Check sheet for the modelled part. Datum: model origin and axes. Units: mm. A direction names the side the tool comes from. Coordinates: 2 decimals unless noted, no trailing zeros. Loops run counter-clockwise (first coordinate to the right, second up) from the corner with the lowest first, then second, coordinate; pieces in that order, holes last. Notation, with made-up numbers: (0, 11) - (58, 11) arc R31 ccw to (58, 38) - close; hole circle Ø5 at (87, -0.5). An arc over 180 degrees is marked (long way). Write each question's results on one line, items separated by ' | '. Start each with the question number.
1. Cross-section at A-A (y = 8.5). Record the cut outline in (x, z), and give its area (3 significant figures).
2. Tool access check on faces 4 (the face through (6, 13, 9)), 5 (the face through (-2.82, -5.02, 8.87)), 6 (the face through (-6, 17.7, 9)), 7 (the face through (-16.55, -5.52, 3.96)). Record the directions out of +Z, -Z, +X, -X, +Y, -Y that give a thin tool (end or side, any length) a straight path to the whole face; none if there is none.
3. Draft check along X on faces 1 (the face through (0, -4.796, 9)), 2 (the face through (-7.16, 9.726, 8.874)), 3 (the face through (-4.808, 0, 9)). Enter one of: released by +X, released by -X, zero draft, split by the parting line, or undercut.
4. Cross-section at B-B (x = 5). Record the cut outline in (y, z), and give its area (3 significant figures).
5. Gauge pin test, flat ends, axial feed: P1, Ø4, axis at y = -0.7, z = 5.25, coming from the +X side; P2, Ø1.5, axis at y = -5, z = 2.5, coming from the +X side; P3, Ø3, axis at y = -6.7, z = 5.25, coming from the -X side. Record the tip position at first contact, or that the pin passes through.
6. Thickness scan on line 1 (Y direction, x = -15.5, z = 5.25); line 2 (X direction, y = -5.5, z = 2); line 3 (Y direction, x = -5.25, z = 2.75). Record the ranges inside material, lowest first. Write a range as [from, to].
```python
from build123d import *

# Parameters (mm, degrees)
BOSS_EXTRUDE1_DEPTH = 18
SKETCH2_R           = 1.75
CUT_EXTRUDE1_DEPTH  = 7


with BuildPart() as part:
    # Sketch1 → Boss-Extrude1 (new body)
    with BuildSketch(Plane.XY):
        with BuildLine():
            Line((7.941784918, -13), (7.941784918, -17.7))
            Line((7.941784918, -17.7), (-20, -17.7))
            Line((-20, -17.7), (-20, 17.699847501))
            Line((-20, 17.699847501), (7.941784918, 17.699847501))
            Line((7.941784918, 17.699847501), (7.941784918, 13))
            Line((7.941784918, 13), (6.333126718, 13))
            Line((6.333126718, 13), (5.317126718, 13))
            Line((5.317126718, 13), (4.287512407, 13))
            ThreePointArc((4.287512407, 13), (3.333616586, 12.604883414), (2.9385, 11.650987593))
            Line((2.9385, 11.650987593), (2.9385, 11.539212407))
            ThreePointArc((2.9385, 11.539212407), (3.333616586, 10.585316586), (4.287512407, 10.1902))
            Line((4.287512407, 10.1902), (6.476788598, 10.1902))
            ThreePointArc((6.476788598, 10.1902), (7.154992901, 9.736757749), (6.995146796, 8.93674514))
            Line((6.995146796, 8.93674514), (3.686383353, 5.635543623))
            ThreePointArc((3.686383353, 5.635543623), (2.754473742, 5.014017446), (1.655778399, 4.7958))
            Line((1.655778399, 4.7958), (-1.655778399, 4.7958))
            ThreePointArc((-1.655778399, 4.7958), (-2.754473742, 5.014017446), (-3.686383353, 5.635543623))
            Line((-3.686383353, 5.635543623), (-6.995146796, 8.93674514))
            ThreePointArc((-6.995146796, 8.93674514), (-7.154992901, 9.736757749), (-6.476788598, 10.1902))
            Line((-6.476788598, 10.1902), (-4.287512407, 10.1902))
            ThreePointArc((-4.287512407, 10.1902), (-3.333616586, 10.585316586), (-2.9385, 11.539212407))
            Line((-2.9385, 11.539212407), (-2.9385, 11.650987593))
            ThreePointArc((-2.9385, 11.650987593), (-3.333616586, 12.604883414), (-4.287512407, 13))
            Line((-4.287512407, 13), (-5.317126718, 13))
            Line((-5.317126718, 13), (-6.333126718, 13))
            Line((-6.333126718, 13), (-9.550465633, 13))
            Line((-9.550465633, 13), (-10.564722121, 12.999847763))
            ThreePointArc((-10.564722121, 12.999847763), (-12.294654751, 12.29465435), (-12.999847757, 10.564721553))
            Line((-12.999847757, 10.564721553), (-13, 9.550422515))
            Line((-13, 9.550422515), (-13, 5.3170836))
            Line((-13, 5.3170836), (-13, 4.287469289))
            ThreePointArc((-13, 4.287469289), (-12.604883414, 3.333573468), (-11.650987593, 2.938456882))
            Line((-11.650987593, 2.938456882), (-11.539212407, 2.938456882))
            ThreePointArc((-11.539212407, 2.938456882), (-10.585316586, 3.333573468), (-10.1902, 4.287469289))
            Line((-10.1902, 4.287469289), (-10.1902, 6.402089023))
            ThreePointArc((-10.1902, 6.402089023), (-9.74154152, 7.073969797), (-8.94902056, 6.917034355))
            Line((-8.94902056, 6.917034355), (-5.652895046, 3.628441884))
            ThreePointArc((-5.652895046, 3.628441884), (-5.027976112, 2.694919539), (-4.8085, 1.593185507))
            Line((-4.8085, 1.593185507), (-4.8085, -1.593185507))
            ThreePointArc((-4.8085, -1.593185507), (-5.027976112, -2.694919539), (-5.652895046, -3.628441884))
            Line((-5.652895046, -3.628441884), (-8.94902056, -6.917034355))
            ThreePointArc((-8.94902056, -6.917034355), (-9.74154152, -7.073969797), (-10.1902, -6.402089023))
            Line((-10.1902, -6.402089023), (-10.1902, -4.287469289))
            ThreePointArc((-10.1902, -4.287469289), (-10.585316586, -3.333573468), (-11.539212407, -2.938456882))
            Line((-11.539212407, -2.938456882), (-11.650987593, -2.938456882))
            ThreePointArc((-11.650987593, -2.938456882), (-12.604883414, -3.333573468), (-13, -4.287469289))
            Line((-13, -4.287469289), (-13, -5.3170836))
            Line((-13, -5.3170836), (-13, -6.3330836))
            Line((-13, -6.3330836), (-13, -9.550422515))
            Line((-13, -9.550422515), (-12.999847757, -10.564721553))
            ThreePointArc((-12.999847757, -10.564721553), (-12.294654751, -12.29465435), (-10.564722121, -12.999847763))
            Line((-10.564722121, -12.999847763), (-9.550465633, -13))
            Line((-9.550465633, -13), (-6.333126718, -13))
            Line((-6.333126718, -13), (-5.317126718, -13))
            Line((-5.317126718, -13), (-4.287512407, -13))
            ThreePointArc((-4.287512407, -13), (-3.333616586, -12.604883414), (-2.9385, -11.650987593))
            Line((-2.9385, -11.650987593), (-2.9385, -11.539212407))
            ThreePointArc((-2.9385, -11.539212407), (-3.333616586, -10.585316586), (-4.287512407, -10.1902))
            Line((-4.287512407, -10.1902), (-6.416408329, -10.1902))
            ThreePointArc((-6.416408329, -10.1902), (-7.137514675, -9.708134418), (-6.967711912, -8.857517813))
            Line((-6.967711912, -8.857517813), (-3.740331666, -5.636015806))
            ThreePointArc((-3.740331666, -5.636015806), (-2.808257752, -5.01414519), (-1.709253557, -4.7958))
            Line((-1.709253557, -4.7958), (1.709253557, -4.7958))
            ThreePointArc((1.709253557, -4.7958), (2.808257752, -5.01414519), (3.740331666, -5.636015806))
            Line((3.740331666, -5.636015806), (6.967711912, -8.857517813))
            ThreePointArc((6.967711912, -8.857517813), (7.137514675, -9.708134418), (6.416408329, -10.1902))
            Line((6.416408329, -10.1902), (4.287512407, -10.1902))
            ThreePointArc((4.287512407, -10.1902), (3.333616586, -10.585316586), (2.9385, -11.539212407))
            Line((2.9385, -11.539212407), (2.9385, -11.650987593))
            ThreePointArc((2.9385, -11.650987593), (3.333616586, -12.604883414), (4.287512407, -13))
            Line((4.287512407, -13), (5.317126718, -13))
            Line((5.317126718, -13), (6.333126718, -13))
            Line((6.333126718, -13), (7.941784918, -13))
        make_face()
    extrude(amount=BOSS_EXTRUDE1_DEPTH)

    # Sketch2 → Cut-Extrude1 (cut)
    with BuildSketch(Plane.ZY.offset(20)):
        with Locations((5.25, -0.7)):
            Circle(SKETCH2_R)
        with Locations((12.75, -0.7)):
            Circle(SKETCH2_R)
        with Locations((5.25, -6.7)):
            Circle(SKETCH2_R)
        with Locations((12.75, -6.7)):
            Circle(SKETCH2_R)
    extrude(amount=-CUT_EXTRUDE1_DEPTH, mode=Mode.SUBTRACT)


solid = part.part
```
Established:
1) outline: (-20, 0) - (-13, 0) - (-13, 18) - (-20, 18) - close; (-6.56, 0) - (6.56, 0) - (6.56, 18) - (-6.56, 18) - close | area: 362 mm^2
2) face 4: +Z, -Z, +X | face 5: +Z, -Z | face 6: +Z, -Z, +X, -X, +Y | face 7: -X
3) face 1: zero draft | face 2: undercut | face 3: released by +X
4) outline: (-17.7, 0) - (-13, 0) - (-13, 18) - (-17.7, 18) - close; (-10.19, 0) - (-6.89, 0) - (-6.89, 18) - (-10.19, 18) - close; (6.95, 0) - (10.19, 0) - (10.19, 18) - (6.95, 18) - close; (13, 0) - (17.7, 0) - (17.7, 18) - (13, 18) - close | area: 287 mm^2
5) P1: x = -4.81 | P2: x = 3.85 | P3: x = -10.19
6) line 1: [-17.7, -8.45], [-4.95, -2.45], [1.05, 17.7] | line 2: [-20, -13], [-10.19, -7.53], [-3.59, 3.59] | line 3: [-17.7, -13], [-10.19, -7.14], [-3.12, 3.12], [7.2, 10.19], [13, 17.7]
